Geometry: final body of the model. Coordinates: model frame, mm. A direction names the side the tool comes from. Give positions to 0.01 mm unless a question says otherwise; leave off trailing zeros. Order: outer loops, then holes, each group sorted by start corner. A loop starts at its lowest first (then second) coordinate and runs counter-clockwise, first axis right, second up. Notation, with made-up numbers: (85, -21.5) - (110, -21.5) arc R19 ccw to (110, 4.5) - close; hole circle Ø11 at (28, 17.5). An arc over 180 degrees is marked (long way). One line per item, written item: value.
```python
from build123d import *

# Parameters (mm, degrees)
SKETCH_1_W          = 24.5
SKETCH_1_H          = 38
EXTRUDE_1_DEPTH     = 2
SKETCH_4_R          = 2.05
CUT_EXTRUDE_1_DEPTH = 1
SKETCH_9_R          = 1
CUT_EXTRUDE_3_DEPTH = 1
CUT_EXTRUDE_4_REACH = 146.905
SKETCH_10_R         = 0.5
FILLET_1_R          = 1
SKETCH_11_W         = 5.762947655
SKETCH_11_H         = 2.6557086
EXTRUDE_2_DEPTH     = 5
SKETCH_12_W         = 8
SKETCH_12_H         = 1.496173859
EXTRUDE_3_DEPTH     = 5


with BuildPart() as part:
    # Sketch 1 → Extrude 1 (new body)
    with BuildSketch(Plane.XY):
        with Locations((-110.040086771, 58.72858385)):
            Rectangle(SKETCH_1_W, SKETCH_1_H)
    extrude(amount=EXTRUDE_1_DEPTH)

    # Sketch 4 → Cut-Extrude 1 (cut)
    with BuildSketch(Plane(origin=(0, 0, 0), x_dir=(-1, 0, 0), z_dir=(0, 0, -1))):
        with Locations((118.450086771, 67.72858385)):
            Circle(SKETCH_4_R)
    extrude(amount=-CUT_EXTRUDE_1_DEPTH, mode=Mode.SUBTRACT)

    # Sketch 9 → Cut-Extrude 3 (cut)
    with BuildSketch(Plane.XY.offset(2)):
        with Locations((-99.090086771, 76.42858385)):
            Circle(SKETCH_9_R)
        with Locations((-99.090086771, 41.02858385)):
            Circle(SKETCH_9_R)
        with Locations((-120.990086771, 41.02858385)):
            Circle(SKETCH_9_R)
        with Locations((-120.990086771, 76.42858385)):
            Circle(SKETCH_9_R)
    extrude(amount=-CUT_EXTRUDE_3_DEPTH, mode=Mode.SUBTRACT)

    # Sketch 10 → Cut-Extrude 4 (cut, up to next)
    with BuildSketch(Plane.XY.offset(1), mode=Mode.PRIVATE) as cut_extrude_4_sk1:
        with Locations((-120.990086771, 41.02858385)):
            Circle(SKETCH_10_R)
    cut_extrude_4_tool1 = extrude(cut_extrude_4_sk1.sketch, amount=-CUT_EXTRUDE_4_REACH, mode=Mode.PRIVATE) & part.part
    # Sketch 10 → Cut-Extrude 4 (cut, up to next)
    with BuildSketch(Plane.XY.offset(1), mode=Mode.PRIVATE) as cut_extrude_4_sk2:
        with Locations((-99.090086771, 41.02858385)):
            Circle(SKETCH_10_R)
    cut_extrude_4_tool2 = extrude(cut_extrude_4_sk2.sketch, amount=-CUT_EXTRUDE_4_REACH, mode=Mode.PRIVATE) & part.part
    # Sketch 10 → Cut-Extrude 4 (cut, up to next)
    with BuildSketch(Plane.XY.offset(1), mode=Mode.PRIVATE) as cut_extrude_4_sk3:
        with Locations((-99.090086771, 76.42858385)):
            Circle(SKETCH_10_R)
    cut_extrude_4_tool3 = extrude(cut_extrude_4_sk3.sketch, amount=-CUT_EXTRUDE_4_REACH, mode=Mode.PRIVATE) & part.part
    # Sketch 10 → Cut-Extrude 4 (cut, up to next)
    with BuildSketch(Plane.XY.offset(1), mode=Mode.PRIVATE) as cut_extrude_4_sk4:
        with Locations((-120.990086771, 76.42858385)):
            Circle(SKETCH_10_R)
    cut_extrude_4_tool4 = extrude(cut_extrude_4_sk4.sketch, amount=-CUT_EXTRUDE_4_REACH, mode=Mode.PRIVATE) & part.part
    add(cut_extrude_4_tool1.solids().sort_by_distance((-120.990087, 41.028584, 1))[0], mode=Mode.SUBTRACT)
    add(cut_extrude_4_tool2.solids().sort_by_distance((-99.090087, 41.028584, 1))[0], mode=Mode.SUBTRACT)
    add(cut_extrude_4_tool3.solids().sort_by_distance((-99.090087, 76.428584, 1))[0], mode=Mode.SUBTRACT)
    add(cut_extrude_4_tool4.solids().sort_by_distance((-120.990087, 76.428584, 1))[0], mode=Mode.SUBTRACT)

    # Fillet 1
    fillet_1_edges = [part.edges().sort_by_distance(p)[0] for p in [
        (-97.790086771, 39.72858385, 1),
        (-122.290086771, 39.72858385, 1),
        (-122.290086771, 77.72858385, 1),
        (-97.790086771, 77.72858385, 1),
    ]]
    fillet(fillet_1_edges, radius=FILLET_1_R)

    # Sketch 11 → Extrude 2 (add)
    with BuildSketch(Plane(origin=(0, 0, 0), x_dir=(-1, 0, 0), z_dir=(0, 0, -1))):
        with Locations((108.208612944, 65.75072955)):
            Rectangle(SKETCH_11_W, SKETCH_11_H)
    extrude(amount=EXTRUDE_2_DEPTH)

    # Sketch 12 → Extrude 3 (add)
    with BuildSketch(Plane(origin=(0, 0, 0), x_dir=(-1, 0, 0), z_dir=(0, 0, -1))):
        with Locations((110.636291242, 49.77667078)):
            Rectangle(SKETCH_12_W, SKETCH_12_H)
    extrude(amount=EXTRUDE_3_DEPTH)


solid = part.part
```
1) Section C-C, the plane x = -109. Return loops of the section in (y, z).
Answers below:
outline: (39.73, 0) - (49.03, 0) - (49.03, -5) - (50.52, -5) - (50.52, 0) - (64.42, 0) - (64.42, -5) - (67.08, -5) - (67.08, 0) - (77.73, 0) - (77.73, 2) - (39.73, 2) - close
2) First-contact query: pin 1 (1.3 mm diameter, centred on y = 66, z = -1.5, fed in from +X); pin 2 (3 mm diameter, centred on y = 66.5, z = -3.5, fed in from -X); pin 3 (1.5 mm diameter, centred on y = 56, z = -1, fed in from +X); pin 4 (3 mm diameter, centred on x = -108, z = -3.5, fed in from +Y). Flat tips, straight axial feed; report the tip coordinate or a pass-through.
Answers below:
pin 1: x = -105.33
pin 2: x = -111.09
pin 3: through
pin 4: y = 67.08
3) Section A-A, the plane z = -1.5. Return loops of the section in (x, y).
Answers below:
outline: (-114.64, 49.03) - (-106.64, 49.03) - (-106.64, 50.52) - (-114.64, 50.52) - close; (-111.09, 64.42) - (-105.33, 64.42) - (-105.33, 67.08) - (-111.09, 67.08) - close
4) Material intervals for line 1 along Z through (x, y) = (-108.25, 43); line 2 along Y through (x, z) = (-111.25, -2.5), sorted ascending.
Answers below:
line 1: 0 to 2
line 2: 49.03 to 50.52
5) Section D-D, the plane x = -111.75. Return loops of the section in (y, z), then the cut area to 3 significant figures.
Answers below:
outline: (39.73, 0) - (49.03, 0) - (49.03, -5) - (50.52, -5) - (50.52, 0) - (77.73, 0) - (77.73, 2) - (39.73, 2) - close
area: 83.5 mm^2
6) Set-up query: faces 1 (the face through (-106.636, 50, -2)), 2 (the face through (-111, 50.525, -2)), 3 (the face through (-111, 49.029, -2)), 4 (the face through (-99.884, 75.82, 1.507)), 5 (the face through (-114.636, 50, -2)). Return all of +Z, -Z, +X, -X, +Y, -Y with unobstructed straight access to the full face (end or side cutting, diameter ignored); none if empty.
Answers below:
face 1: -Z, +X, -Y
face 2: -Z, +X, -X
face 3: -Z, +X, -X, -Y
face 4: +Z
face 5: -Z, -X, +Y, -Y
7) Section B-B, the plane y = 49.5. Return loops of the section in (x, z), then the cut area to 3 significant figures.
Answers below:
outline: (-122.29, 0) - (-114.64, 0) - (-114.64, -5) - (-106.64, -5) - (-106.64, 0) - (-97.79, 0) - (-97.79, 2) - (-122.29, 2) - close
area: 89.0 mm^2
